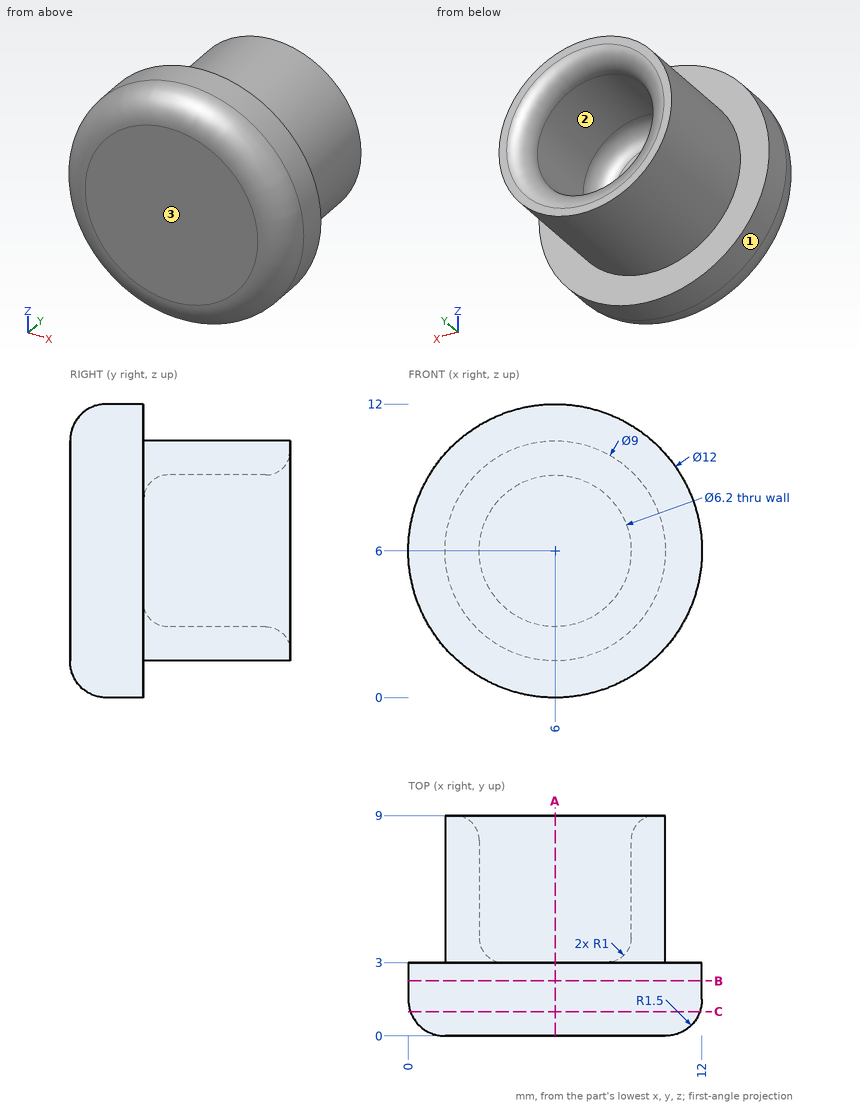
Job drawing, mm, ordinate dimensions from the low corner. One solid piece. Coordinates: 2 decimals unless noted, no trailing zeros. Write each loop counter-clockwise with the first axis right and the second up, starting at its lowest first coordinate (ties: lowest second). Pieces come first, ordered by that corner, then holes. Notation, with made-up numbers: (-16, 83.25) - (27, 83.25) arc R26 cw to (27, 99.25) - close; hole circle Ø9 at (15, 10). An arc over 180 degrees is marked (long way). Use a Markdown table: item, result. Add a question column.
Item 1: Flat gauge pins, fed straight in: pin 1 (1.5 mm diameter, centred on y = 7, z = 5.5, fed in from +X); pin 2 (1 mm diameter, centred on y = 7.5, z = 2.5, fed in from +X); pin 3 (6 mm diameter, centred on x = 8.5, z = 7, fed in from +Y); pin 4 (1.3 mm diameter, centred on x = 6, z = 5.5, fed in from +Y). Where does each tip first touch, or does it go through?
Item 2: Mould opens along Z. For the marked faces 1, 2 and 3 say: pulls with the +Z half, pulls with the -Z half, needs draft (parallel to the pull), parting line crosses it, or undercut.
Item 3: Drill centre lines: L1, parallel to Z at x = 6, y = 4.95; L2, parallel to X at y = 7.5, z = 3.25; L3, parallel to X at y = 5.5, z = 4.25. Where is each one in solid material? Low to high. Write a range as from..to.
Item 4: Band-saw the part on A-A, the plane x = 6. Give the cut face in (y, z), and give its area (3 significant figures).
Item 5: Band-saw the part on C-C, the plane y = 1. Give the cut face in (x, z).
Item 6: Band-saw the part on B-B, the plane y = 2.25. Give the cut face in (x, z), and give its area (3 significant figures).
Numbers:
| question | item | result |
|---|---|---|
| 1 | pin 1 | x = 10.5 |
| 1 | pin 2 | x = 9.35 |
| 1 | pin 3 | y = 9 |
| 1 | pin 4 | y = 3 |
| 2 | face 1 | parting line crosses it |
| 2 | face 2 | undercut |
| 2 | face 3 | needs draft |
| 3 | L1 | 1.5..2.9, 9.1..10.5 |
| 3 | L2 | 2.44..4.57, 7.43..9.56 |
| 3 | L3 | 1.85..3.44, 8.56..10.15 |
| 4 | outline | (0, 1.5) arc R1.5 ccw to (1.5, 0) - (3, 0) - (3, 1.5) - (9, 1.5) - (9, 1.9) arc R1 ccw to (8, 2.9) - (4, 2.9) arc R1 cw to (3, 3.9) - (3, 8.1) arc R1 cw to (4, 9.1) - (8, 9.1) arc R1 ccw to (9, 10.1) - (9, 10.5) - (3, 10.5) - (3, 12) - (1.5, 12) arc R1.5 ccw to (0, 10.5) - close |
| 4 | area | 51.8 mm2 |
| 5 | outline | circle Ø11.83 at (6, 6) |
| 6 | outline | circle Ø12 at (6, 6) |
| 6 | area | 113 mm2 |
